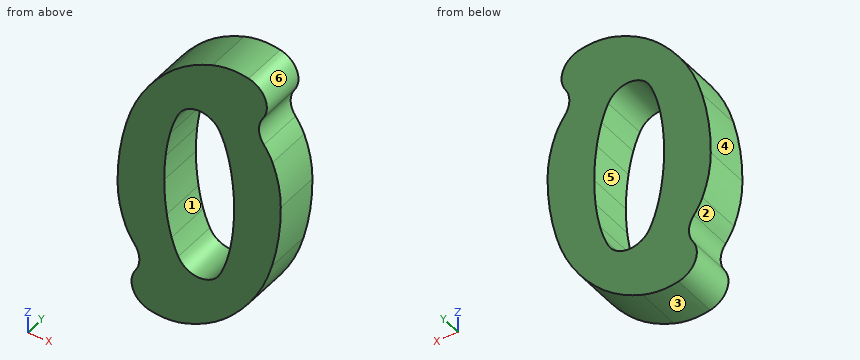
```python
from build123d import *

# Parameters (mm, degrees)
F1_DEPTH = 12.7


# Not quite as in the source:
# - ends of sketch curves that miss each other by under 0.0002 mm in the source are joined


with BuildPart() as f1:
    # F0 (on Front) → F1 (new body)
    with BuildSketch(Plane.XZ):
        with BuildLine():
            ThreePointArc((303.2931532121, 303.0067577098), (301.4715319233, 294.1610584771), (300.8818774244, 285.1490106185))
            ThreePointArc((300.8818774244, 285.1490106185), (301.4449295055, 279.0945065847), (303.1390906491, 273.2546565343))
            ThreePointArc((303.1390906491, 273.2546565343), (304.1794047627, 271.163745604), (305.4871188741, 269.2287914427))
            ThreePointArc((305.4871188741, 269.2287914427), (306.8191261994, 265.559271793), (305.752743748, 261.8039536514))
            ThreePointArc((305.752743748, 261.8039536514), (305.1400456304, 255.9083712227), (309.6612562028, 252.0753703346))
            ThreePointArc((309.6612562028, 252.0753703346), (314.6118369552, 251.6558987634), (319.4911798503, 252.5919579373))
            ThreePointArc((319.4911798503, 252.5919579373), (326.238452414, 255.7664937708), (332.0491509461, 260.4397327714))
            ThreePointArc((332.0491509461, 260.4397327714), (338.7629233679, 269.1816350422), (342.9782332171, 279.3662684747))
            ThreePointArc((342.9782332171, 279.3662684747), (344.8007217874, 288.2183656036), (345.3891604556, 297.2369467464))
            ThreePointArc((345.3891604556, 297.2369467464), (344.8270625572, 303.274887915), (343.1402655074, 309.0996131302))
            ThreePointArc((343.1402655074, 309.0996131302), (342.0995588503, 311.1979660981), (340.7875354527, 313.1382632658))
            ThreePointArc((340.7875354527, 313.1382632658), (339.4517460358, 316.8098548296), (340.5182976713, 320.568494544))
            ThreePointArc((340.5182976713, 320.568494544), (341.1313810425, 326.4642550769), (336.610094213, 330.2975007104))
            ThreePointArc((336.610094213, 330.2975007104), (331.659512348, 330.7170042507), (326.7801614181, 329.7809489664))
            ThreePointArc((326.7801614181, 329.7809489664), (320.0328916386, 326.6063773725), (314.2221892806, 321.9331298991))
            ThreePointArc((314.2221892806, 321.9331298991), (307.5084491355, 313.1913079367), (303.2931532121, 303.0067577098))
        make_face()
        with BuildLine():
            ThreePointArc((315.1713123146, 305.1180818659), (315.8393495072, 307.515035294), (316.678097317, 309.857717846))
            ThreePointArc((316.678097317, 309.857717846), (317.0633180741, 310.7621499557), (317.4920222134, 311.6467997261))
            ThreePointArc((317.4920222134, 311.6467997261), (323.2069159103, 315.0891849126), (328.8450890708, 311.5225170196))
            ThreePointArc((328.8450890708, 311.5225170196), (329.8473834441, 309.2127575845), (330.6417253346, 306.8234892773))
            ThreePointArc((330.6417253346, 306.8234892773), (331.4003540176, 303.8138045335), (331.9581118177, 300.7605072271))
            ThreePointArc((331.9581118177, 300.7605072271), (332.4883254582, 295.994995702), (332.6606828218, 291.2031767897))
            ThreePointArc((332.6606828218, 291.2031767897), (332.5693501994, 287.6782798164), (332.2892894077, 284.1633395865))
            ThreePointArc((332.2892894077, 284.1633395865), (331.8093085942, 280.6893291587), (331.1000077041, 277.2547960368))
            ThreePointArc((331.1000077041, 277.2547960368), (330.4319997673, 274.8578337912), (329.5932507917, 272.5151498081))
            ThreePointArc((329.5932507917, 272.5151498081), (329.2080362587, 271.6107324514), (328.7793397252, 270.7260967499))
            ThreePointArc((328.7793397252, 270.7260967499), (323.064427394, 267.2836913001), (317.4262371292, 270.8503593804))
            ThreePointArc((317.4262371292, 270.8503593804), (316.4239511956, 273.1601221417), (315.6296075412, 275.5493890189))
            ThreePointArc((315.6296075412, 275.5493890189), (314.8709725785, 278.5590700417), (314.3132149314, 281.612365479))
            ThreePointArc((314.3132149314, 281.612365479), (313.7830008793, 286.3778788276), (313.6106433782, 291.1696996103))
            ThreePointArc((313.6106433782, 291.1696996103), (313.7020014012, 294.6945965951), (313.9820621923, 298.2095368135))
            ThreePointArc((313.9820621923, 298.2095368135), (314.4620178297, 301.6835485419), (315.1713123146, 305.1180818659))
        make_face(mode=Mode.SUBTRACT)
    extrude(amount=F1_DEPTH)


solid = f1.part
```
Design review of the part built by this model. Coordinates are the model's own, in mm. Face numbers are marked on the shaded views. A direction names the side the tool comes from. Give positions to 0.01 mm unless a question says otherwise; leave off trailing zeros. Order: outer loops, then holes, each group sorted by start corner. A loop starts at its lowest first (then second) coordinate and runs counter-clockwise, first axis right, second up. Notation, with made-up numbers: (29.25, 80) - (66.25, 80) arc R16 ccw to (66.25, 105) - close; hole circle Ø3 at (71, 55). An arc over 180 degrees is marked (long way). Use a Markdown table: item, result. Add a question column.
(1) Add section A-A on z = 287. Give the boundary of the cut face in (x, y).
(2) Machinability: for the marked faces 1, 2 and 3, which of the approach directions +Z, -Z, +X, -X, +Y, -Y give a long, thin tool a straight path to every point of the face, cutting with its end or side? Answer none if there is none.
(3) Add section C-C on x = 324. Give the boundary of the cut face in (y, z), then the cut area to 3 significant figures.
(4) Mouldability with a two-part tool opening along X and no side actions: class the marked faces 4, 5 and 6 as +X half, -X half, draft (parallel to the pull), parting line (faces both ways), or undercut.
(5) Wall thickness on probe 1 along X at (y, z) = (-1.5, 295); probe 2 along X at (y, z) = (-8.5, 276.5); probe 3 along Z at (x, y) = (320, -5.5): over which ranges is each line inside the solid? List them lowest first. Write a range as [from, to].
(6) Add section D-D on x = 312.5. Give the boundary of the cut face in (y, z).
(7) Clearance check with flat-ended pins moving along their axes: P1, Ø6, axis at y = -8.5, z = 262.5, coming from the +X side; P2, Ø4, axis at y = -6.5, z = 303, coming from the +X side; P3, Ø3, axis at y = -2, z = 314.5, coming from the -X side. State where each tip first meets the part, or that it passes through.
Report:
| question | item | result |
|---|---|---|
| 1 | outline | (300.9, -12.7) - (313.74, -12.7) - (313.74, 0) - (300.9, 0) - close; (332.53, -12.7) - (344.62, -12.7) - (344.62, 0) - (332.53, 0) - close |
| 2 | face 1 | +Y, -Y |
| 2 | face 2 | -X, +Y, -Y |
| 2 | face 3 | -Z, +Y, -Y |
| 3 | outline | (-12.7, 254.49) - (0, 254.49) - (0, 267.34) - (-12.7, 267.34) - close; (-12.7, 315.03) - (0, 315.03) - (0, 328.71) - (-12.7, 328.71) - close |
| 3 | area | 337 mm² |
| 4 | face 4 | -X half |
| 4 | face 5 | undercut |
| 4 | face 6 | +X half |
| 5 | probe 1 | x = [301.59, 313.72], [332.55, 345.36] |
| 5 | probe 2 | x = [302.05, 315.37], [330.91, 342.1] |
| 5 | probe 3 | z = [252.77, 268.11], [314.26, 326.59] |
| 6 | outline | (-12.7, 251.67) - (0, 251.67) - (0, 320.11) - (-12.7, 320.11) - close |
| 7 | P1 | stops at x = 336.37 |
| 7 | P2 | stops at x = 345.17 |
| 7 | P3 | stops at x = 307.4 |
